Work out the finished part from the listing and answer in its coordinate system (mm). Face numbers are marked on the shaded views. A direction names the side the tool comes from. Round coordinates to 2 decimals unless told otherwise and drop trailing zeros. Order: outer loops, then holes, each group sorted by start corner. A loop starts at its lowest first (then second) coordinate and runs counter-clockwise, first axis right, second up. Notation, with made-up numbers: (-31, 46) - (21, 46) arc R16 ccw to (21, 72) - close; hole circle Ø9 at (-6, 4.5). An arc over 180 degrees is marked (long way). Answer in a Markdown table with one row per item.
from build123d import *

# Parameters (mm, degrees)
F0_W      = 90
F0_H      = 52
F0_R      = 1.65
F0_R_2    = 7.5
F0_W_2    = 2.5
F0_H_2    = 10
F1_DEPTH  = 4
F2_DEPTH  = 3
F3_W      = 90
F3_H      = 5
F4_DEPTH  = 55
F5_W      = 15.3
F5_H      = 1
F6_DEPTH  = 15
F7_R      = 1.65
F8_DEPTH  = 3
F9_R      = 1.65
F10_DEPTH = 5
F11_R     = 3.25
F12_DEPTH = 3
F14_DEPTH = 2
F16_DEPTH = 3
F17_DEPTH = 20
F18_R     = 2.15
F19_DEPTH = 3
F20_R     = 1.65
F21_DEPTH = 2.6730195726
F22_R     = 1.65
F23_DEPTH = 3
F24_R     = 1
F25_R     = 5


# Not quite as in the source:
# - a pattern or mirror of a feature is missing from the dataset's text; its kind, count and spacing are read off the source's solid
# - a feature names something its author has since deleted; it is built from what else it names


with BuildPart() as f1:
    # F0 (on Top) → F1 (new body)
    with BuildSketch(Plane.XY):
        with Locations((0, -8.8)):
            Rectangle(F0_W, F0_H)
        with BuildLine():
            ThreePointArc((-19.5, -32.45), (-21.15, -30.8), (-19.5, -29.15))
            Line((-19.5, -29.15), (-11.5, -29.15))
            ThreePointArc((-11.5, -29.15), (-10.333273811, -29.633273811), (-9.85, -30.8))
            ThreePointArc((-9.85, -30.8), (-10.333273811, -31.966726189), (-11.5, -32.45))
            Line((-11.5, -32.45), (-19.5, -32.45))
        make_face(mode=Mode.SUBTRACT)
        with BuildLine():
            ThreePointArc((19.5, -29.15), (20.666726189, -29.633273811), (21.15, -30.8))
            ThreePointArc((21.15, -30.8), (20.666726189, -31.966726189), (19.5, -32.45))
            Line((19.5, -32.45), (11.5, -32.45))
            ThreePointArc((11.5, -32.45), (9.85, -30.8), (11.5, -29.15))
            Line((11.5, -29.15), (19.5, -29.15))
        make_face(mode=Mode.SUBTRACT)
        Polygon((-35, -2), (-35, -12), (35, -12), (35, -2), (37.5, -2), (37.5, -12), (37.5, -14.5), (37.5, -26.5), (-37.5, -26.5), (-37.5, -14.5), (-37.5, -12), (-37.5, -2), align=None, mode=Mode.SUBTRACT)
        with Locations((-42, -5)):
            Circle(F0_R, mode=Mode.SUBTRACT)
        with Locations((-25, 0)):
            Circle(F0_R, mode=Mode.SUBTRACT)
        with Locations((-15, 0)):
            Circle(F0_R, mode=Mode.SUBTRACT)
        with Locations((-42, 5)):
            Circle(F0_R, mode=Mode.SUBTRACT)
        Circle(F0_R_2, mode=Mode.SUBTRACT)
        with Locations((15, 0)):
            Circle(F0_R, mode=Mode.SUBTRACT)
        with Locations((42, -5)):
            Circle(F0_R, mode=Mode.SUBTRACT)
        with Locations((25, 0)):
            Circle(F0_R, mode=Mode.SUBTRACT)
        with Locations((42, 5)):
            Circle(F0_R, mode=Mode.SUBTRACT)
        Polygon((35, -12), (-35, -12), (-37.5, -12), (-37.5, -14.5), (37.5, -14.5), (37.5, -12), align=None)
        with Locations((-36.25, -7)):
            Rectangle(F0_W_2, F0_H_2)
        with Locations((36.25, -7)):
            Rectangle(F0_W_2, F0_H_2)
    extrude(amount=F1_DEPTH)

    # F0 (on Top) → F2 (join)
    with BuildSketch(Plane.XY):
        with Locations((-36.25, -7)):
            Rectangle(F0_W_2, F0_H_2)
        with Locations((36.25, -7)):
            Rectangle(F0_W_2, F0_H_2)
    extrude(amount=F2_DEPTH)

    # F3 (on face) → F4 (join)
    with BuildSketch(Plane.XY.offset(4)):
        with Locations((0, 14.7)):
            Rectangle(F3_W, F3_H)
    extrude(amount=F4_DEPTH)

    # F5 (on face) → F6 (cut)
    with BuildSketch(Plane.XY.offset(59)):
        with Locations((0, 16.7)):
            Rectangle(F5_W, F5_H)
        with Locations((0, 12.7)):
            Rectangle(F5_W, F5_H)
    extrude(amount=-F6_DEPTH, mode=Mode.SUBTRACT)

    # F7 (on face) → F8 (cut, through all)
    with BuildSketch(Plane(origin=(0, 16.2, 0), x_dir=(-1, 0, 0), z_dir=(0, 1, 0))):
        with Locations((0, 51)):
            Circle(F7_R)
    extrude(amount=-F8_DEPTH, mode=Mode.SUBTRACT)

    # F9 (on face) → F10 (cut, through all)
    with BuildSketch(Plane(origin=(0, 17.2, 0), x_dir=(-1, 0, 0), z_dir=(0, 1, 0))):
        with Locations((-40, 17)):
            Circle(F9_R)
        with Locations((-5, 17)):
            Circle(F9_R)
        with Locations((40, 17)):
            Circle(F9_R)
        with Locations((5, 17)):
            Circle(F9_R)
        with Locations((-40, 49)):
            Circle(F9_R)
        with Locations((40, 49)):
            Circle(F9_R)
    extrude(amount=-F10_DEPTH, mode=Mode.SUBTRACT)

    # F11 (on face) → F12 (cut)
    with BuildSketch(Plane.XZ.offset(-12.2)):
        with Locations((5, 17)):
            Circle(F11_R)
        with Locations((40, 17)):
            Circle(F11_R)
        with Locations((-5, 17)):
            Circle(F11_R)
        with Locations((-40, 17)):
            Circle(F11_R)
    extrude(amount=-F12_DEPTH, mode=Mode.SUBTRACT)

    # F13 (on face) → F14 (cut)
    with BuildSketch(Plane.XY):
        with BuildLine():
            ThreePointArc((-22.5, -30.8), (-21.6213203436, -32.9213203436), (-19.5, -33.8))
            Line((-19.5, -33.8), (-11.5, -33.8))
            ThreePointArc((-11.5, -33.8), (-9.3786796564, -32.9213203436), (-8.5, -30.8))
            ThreePointArc((-8.5, -30.8), (-9.3786796564, -28.6786796564), (-11.5, -27.8))
            Line((-11.5, -27.8), (-19.5, -27.8))
            ThreePointArc((-19.5, -27.8), (-21.6213203436, -28.6786796564), (-22.5, -30.8))
        make_face()
        with BuildLine():
            Line((-11.5, -32.45), (-19.5, -32.45))
            ThreePointArc((-19.5, -32.45), (-21.15, -30.8), (-19.5, -29.15))
            Line((-19.5, -29.15), (-11.5, -29.15))
            ThreePointArc((-11.5, -29.15), (-10.333273811, -29.633273811), (-9.85, -30.8))
            ThreePointArc((-9.85, -30.8), (-10.333273811, -31.966726189), (-11.5, -32.45))
        make_face(mode=Mode.SUBTRACT)
        with BuildLine():
            ThreePointArc((8.5, -30.8), (9.3786796564, -32.9213203436), (11.5, -33.8))
            Line((11.5, -33.8), (19.5, -33.8))
            ThreePointArc((19.5, -33.8), (21.6213203436, -32.9213203436), (22.5, -30.8))
            ThreePointArc((22.5, -30.8), (21.6213203436, -28.6786796564), (19.5, -27.8))
            Line((19.5, -27.8), (11.5, -27.8))
            ThreePointArc((11.5, -27.8), (9.3786796564, -28.6786796564), (8.5, -30.8))
        make_face()
        with BuildLine():
            Line((11.5, -29.15), (19.5, -29.15))
            ThreePointArc((19.5, -29.15), (20.666726189, -29.633273811), (21.15, -30.8))
            ThreePointArc((21.15, -30.8), (20.666726189, -31.966726189), (19.5, -32.45))
            Line((19.5, -32.45), (11.5, -32.45))
            ThreePointArc((11.5, -32.45), (9.85, -30.8), (11.5, -29.15))
        make_face(mode=Mode.SUBTRACT)
    extrude(amount=F14_DEPTH, mode=Mode.SUBTRACT)

    # F15 (on face) → F16 (join)
    with BuildSketch(Plane.YZ.offset(45)):
        Polygon((-34.8, 14), (-34.8, 4), (-32.1269804274, 4), (-32.1269804274, 12.6380285008), align=None)
        Polygon((-12.100475013, 58.5503262094), (-34.8, 14), (-32.1269804274, 12.6380285008), (-12.100475013, 51.9422584157), align=None)
        Polygon((-32.1269804274, 12.6380285008), (-32.1269804274, 4), (-12.100475013, 4), (-12.100475013, 51.9422584157), align=None)
    f16 = extrude(amount=-F16_DEPTH)

    # F16_copies: F16 across plane
    add(f16.mirror(Plane(origin=(0, 0, 0), x_dir=(0, 0, -1), z_dir=(-1, 0, 0))))

    # F15 (on face) → F17 (join)
    with BuildSketch(Plane.YZ.offset(45)):
        Polygon((-34.8, 14), (-34.8, 4), (-32.1269804274, 4), (-32.1269804274, 12.6380285008), align=None)
        Polygon((-12.100475013, 58.5503262094), (-34.8, 14), (-32.1269804274, 12.6380285008), (-12.100475013, 51.9422584157), align=None)
    f17 = extrude(amount=-F17_DEPTH)

    # F17_copies: F17 across plane
    add(f17.mirror(Plane(origin=(0, 0, 0), x_dir=(0, 0, -1), z_dir=(-1, 0, 0))))

    # F18 (on face) → F19 (cut, through all)
    with BuildSketch(Plane(origin=(0, -33.2905823505, 16.9623989361), x_dir=(1, 0, 0), z_dir=(0, -0.8910065242, 0.4539904997))):
        with Locations((30, 4.1752219477)):
            Circle(F18_R)
        with Locations((30, 39.1752219477)):
            Circle(F18_R)
    f19 = extrude(amount=-F19_DEPTH, mode=Mode.SUBTRACT)

    # F19_copies: F19 across plane
    add(f19.mirror(Plane(origin=(0, 0, 0), x_dir=(0, 0, -1), z_dir=(-1, 0, 0))), mode=Mode.SUBTRACT)

    # F20 (on face) → F21 (cut, through all)
    with BuildSketch(Plane.XZ.offset(34.8)):
        with Locations((40, 8)):
            Circle(F20_R)
        with Locations((30, 8)):
            Circle(F20_R)
    f21 = extrude(amount=-F21_DEPTH, mode=Mode.SUBTRACT)

    # F21_copies: F21 across plane
    add(f21.mirror(Plane(origin=(0, 0, 0), x_dir=(0, 0, -1), z_dir=(-1, 0, 0))), mode=Mode.SUBTRACT)

    # F22 (on face) → F23 (cut, through all)
    with BuildSketch(Plane.YZ.offset(45)):
        with Locations((-28.4502375065, 8)):
            Circle(F22_R)
        with Locations((-18.4502375065, 8)):
            Circle(F22_R)
        with Locations((-18.4502375065, 18)):
            Circle(F22_R)
        with Locations((-18.4502375065, 28)):
            Circle(F22_R)
    f23 = extrude(amount=-F23_DEPTH, mode=Mode.SUBTRACT)

    # F23_copies: F23 across plane
    add(f23.mirror(Plane(origin=(0, 0, 0), x_dir=(0, 0, -1), z_dir=(-1, 0, 0))), mode=Mode.SUBTRACT)

    # F24
    f24_edges = [f1.edges().sort_by_distance(p)[0] for p in [
        (35, -12.100475, 58.550326),
        (45, -34.8, 7),
        (45, -23.450238, 36.275163),
        (-45, -34.8, 7),
        (-45, -23.450238, 36.275163),
        (-35, -12.100475, 58.550326),
    ]]
    fillet(f24_edges, radius=F24_R)

    # F25
    f25_edges = [f1.edges().sort_by_distance(p)[0] for p in [
        (45, 14.7, 59),
        (-45, 14.7, 59),
        (37.5, -26.5, 2),
        (37.5, -14.5, 2),
        (-37.5, -14.5, 2),
        (-37.5, -26.5, 2),
    ]]
    fillet(f25_edges, radius=F25_R)


solid = f1.part
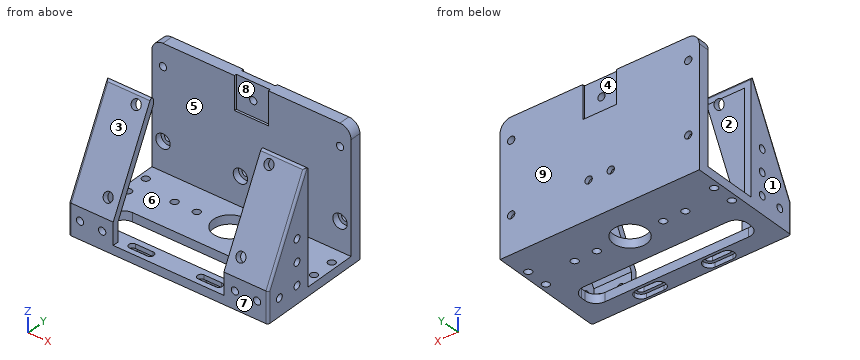
1) Which of the six approach directions +Z, -Z, +X, -X, +Y, -Y give full straight-line access (tool end or side, diameter ignored) to the marked faces 5, 6, 7, 8 and 9?
Filled in:
| item | result |
|---|---|
| face 5 | +Z, +X, -X |
| face 6 | none |
| face 7 | +Z, -Z, +X, -X, -Y |
| face 8 | +Z, -Y |
| face 9 | +Z, -Z, +X, -X, +Y |
2) The mould has two halves that part along X. Classify the marked faces 1, 2, 3 and 4: released by +X, released by -X, zero draft, split by the parting line, or undercut.
Filled in:
| item | result |
|---|---|
| face 1 | released by -X |
| face 2 | undercut |
| face 3 | zero draft |
| face 4 | undercut |
3) Find section A-A, the plane y = 0. Give the vertices of the cut face in (x, z).
Filled in:
| item | result |
|---|---|
| outline | (-45, 0) - (-26.65, 0) - (-26.65, 4) - (-45, 4) - close; (-23.35, 0) - (-16.65, 0) - (-16.65, 4) - (-23.35, 4) - close; (-13.35, 0) - (-7.5, 0) - (-7.5, 4) - (-13.35, 4) - close; (7.5, 0) - (13.35, 0) - (13.35, 4) - (7.5, 4) - close; (16.65, 0) - (23.35, 0) - (23.35, 4) - (16.65, 4) - close; (26.65, 0) - (45, 0) - (45, 4) - (26.65, 4) - close |
4) Find section C-C, the plane x = -5. Give the vertices of the cut face in (y, z), then the cut area to 3 significant figures.
Filled in:
| item | result |
|---|---|
| outline | (-34.8, 0) - (-26.5, 0) - (-26.5, 4) - (-34.8, 4) - close; (-14.5, 0) - (-5.59, 0) - (-5.59, 4) - (-14.5, 4) - close; (5.59, 0) - (17.2, 0) - (17.2, 15.35) - (15.2, 15.35) - (15.2, 13.75) - (12.2, 13.75) - (12.2, 4) - (5.59, 4) - close; (12.2, 20.25) - (15.2, 20.25) - (15.2, 18.65) - (17.2, 18.65) - (17.2, 44) - (16.2, 44) - (16.2, 59) - (13.2, 59) - (13.2, 44) - (12.2, 44) - close |
| area | 334 mm^2 |
5) Find section B-B, the plane z = 8. Give the number of separate pieces and of enclosed holes in the cut face, then the cut area to 3 significant figures.
Filled in:
| item | result |
|---|---|
| separate pieces | 11 |
| enclosed holes | 0 |
| area | 602 mm^2 |
6) Each of these flat-tipped pins is pushed along its axis until it touches: pin 1 (5 mm diameter, centred on x = 28, y = -27, fed in from +Z); pin 2 (6 mm diameter, centred on x = 1.5, z = 43, fed in from -Y); pin 3 (4 mm diameter, centred on x = 22.5, y = -20, fed in from +Z); pin 4 (3 mm diameter, centred on x = -25.5, y = -26.5, fed in from +Z). Where does it stop, or does it pass through?
Filled in:
| item | result |
|---|---|
| pin 1 | stops at z = 34.21 |
| pin 2 | stops at y = 12.2 |
| pin 3 | passes through |
| pin 4 | stops at z = 33.23 |
7) Find the intervals of material crossed by probe 1 along Z at (x, y) = (5, 14); probe 2 along Y at (x, z) = (-3.5, 10); probe 3 along Z at (x, y) = (-17.5, -13.5), in increasing order. Write a range as from..to.
Filled in:
| item | result |
|---|---|
| probe 1 | z = 0..13.75, 20.25..59 |
| probe 2 | y = 12.2..17.2 |
| probe 3 | z = 0..4 |
